Geometry: final body of the model. Coordinates: model frame, mm. A direction names the side the tool comes from. Coordinates: 2 decimals unless noted, no trailing zeros. Loops run counter-clockwise (first coordinate to the right, second up) from the corner with the lowest first, then second, coordinate; pieces in that order, holes last. Notation, with made-up numbers: (30, -15) - (43, -15) arc R17 ccw to (43, -9) - close; hole circle Ø11 at (47.5, 50.25). An arc over 180 degrees is marked (long way). Answer in a Markdown table with one row per item.
from build123d import *

# Parameters (mm, degrees)
ESQUISSE1_W        = 20
ESQUISSE1_H        = 11
BOSS_EXTRU_1_DEPTH = 2
ESQUISSE2_R        = 1
BOSS_EXTRU_2_DEPTH = 3
CONG_1_R           = 1
ESQUISSE3_R        = 1.5
BOSS_EXTRU_3_DEPTH = 2
CONG_2_R           = 2


with BuildPart() as part:
    # Esquisse1 → Boss.-Extru.1 (new body)
    with BuildSketch(Plane.XY):
        with Locations((10, 5.5)):
            Rectangle(ESQUISSE1_W, ESQUISSE1_H)
    extrude(amount=BOSS_EXTRU_1_DEPTH)

    # Esquisse2 → Boss.-Extru.2 (add)
    with BuildSketch(Plane.XY.offset(2)):
        with Locations(Location((16.25, 3, 0), (0, 0, 180))):
            Circle(ESQUISSE2_R)
        with Locations(Location((3.75, 3, 0), (0, 0, 180))):
            Circle(ESQUISSE2_R)
    extrude(amount=BOSS_EXTRU_2_DEPTH)

    # Congé1
    cong_1_edges = [part.edges().sort_by_distance(p)[0] for p in [
        (17.25, 3, 2),
        (4.75, 3, 2),
    ]]
    fillet(cong_1_edges, radius=CONG_1_R)

    # Esquisse3 → Boss.-Extru.3 (add)
    with BuildSketch(Plane(origin=(0, 11, 0), x_dir=(1, 0, 0), z_dir=(0, 1, 0))):
        Polygon((0, 0), (0, -2), (20, -2), (20, 0), (13, 0), (13, 7.5), (7, 7.5), (7, 0), align=None)
        with Locations(Location((10, 4.5, 0), (0, 0, 270))):
            Circle(ESQUISSE3_R, mode=Mode.SUBTRACT)
    extrude(amount=BOSS_EXTRU_3_DEPTH)

    # Congé2
    cong_2_edges = [part.edges().sort_by_distance(p)[0] for p in [
        (7, 12, 0),
        (13, 12, 0),
    ]]
    fillet(cong_2_edges, radius=CONG_2_R)


solid = part.part
(1) Ray query, probe 1 along X at (y, z) = (12.6, -4.5); probe 2 along Y at (x, z) = (8, -4.75); probe 3 along Z at (x, y) = (1, 10.25). Return the intervals inside material, ascending.
Verdict:
| item | result |
|---|---|
| probe 1 | x = 7 to 8.5, 11.5 to 13 |
| probe 2 | y = 11 to 13 |
| probe 3 | z = 0 to 2 |
(2) Cut plane A-A on z = -4.5. Output: boundary loops of the cut face in (x, y), then the cut area to 3 significant figures.
Verdict:
| item | result |
|---|---|
| outline | (7, 11) - (8.5, 11) - (8.5, 13) - (7, 13) - close; (11.5, 11) - (13, 11) - (13, 13) - (11.5, 13) - close |
| area | 6.00 mm² |
(3) Cut plane B-B on y = 3. Output: boundary loops of the cut face in (x, z).
Verdict:
| item | result |
|---|---|
| outline | (0, 0) - (20, 0) - (20, 2) - (18.25, 2) arc R1 cw to (17.25, 3) - (17.25, 5) - (15.25, 5) - (15.25, 3) arc R1 cw to (14.25, 2) - (5.75, 2) arc R1 cw to (4.75, 3) - (4.75, 5) - (2.75, 5) - (2.75, 3) arc R1 cw to (1.75, 2) - (0, 2) - close |
(4) Cut plane C-C on x = 10. Output: boundary loops of the cut face in (y, z).
Verdict:
| item | result |
|---|---|
| outline | (0, 0) - (11, 0) - (11, -3) - (13, -3) - (13, 2) - (0, 2) - close; (11, -7.5) - (13, -7.5) - (13, -6) - (11, -6) - close |
(5) Cut plane D-D on x = 16.25. Output: boundary loops of the cut face in (y, z).
Verdict:
| item | result |
|---|---|
| outline | (0, 0) - (13, 0) - (13, 2) - (5, 2) arc R1 cw to (4, 3) - (4, 5) - (2, 5) - (2, 3) arc R1 cw to (1, 2) - (0, 2) - close |
(6) Access query for faces 4 (the face through (7, 12, -5)), 5 (the face through (9, 11, -3)), 6 (the face through (4.75, 2.96, 3.99)). Directions: +Z, -Z, +X, -X, +Y, -Y. A direction counts if a zero-diameter tool reaches every point of the face in a straight line with its end or side. Return the directions, or none.
Verdict:
| item | result |
|---|---|
| face 4 | -Z, -X, +Y, -Y |
| face 5 | -Z, +X, -X, -Y |
| face 6 | +Z |
(7) First-contact query: pin 1 Ø1 at (y, z) = (12, -5.5) entering from -X; pin 2 Ø0.6 at (y, z) = (12.5, -4.5) entering from +X; pin 3 Ø2.5 at (x, z) = (10, -4.5) entering from -Y. Flat tips, straight axial feed; report the tip coordinate or a pass-through.
Verdict:
| item | result |
|---|---|
| pin 1 | stops at x = 7 |
| pin 2 | stops at x = 13 |
| pin 3 | passes through |
(8) Pull-direction query (Z, two-part tool) for faces 1 (the face through (10, 12, -7.5)), 2 (the face through (8.536, 11.986, -4.825)), 3 (the face through (0, 6, 1)); classes: pulls with the +Z half, pulls with the -Z half, needs draft (parallel to the pull), parting line crosses it, or undercut.
Verdict:
| item | result |
|---|---|
| face 1 | pulls with the -Z half |
| face 2 | undercut |
| face 3 | needs draft |
